Read the model definition and answer for the solid it produces. Units are mm, in the model's axes. Face numbers are marked on the shaded views. A direction names the side the tool comes from. Round coordinates to 2 decimals unless told otherwise and drop trailing zeros. Write each loop counter-clockwise with the first axis right and the second up, starting at its lowest first coordinate (ties: lowest second). Pieces come first, ordered by that corner, then holes.
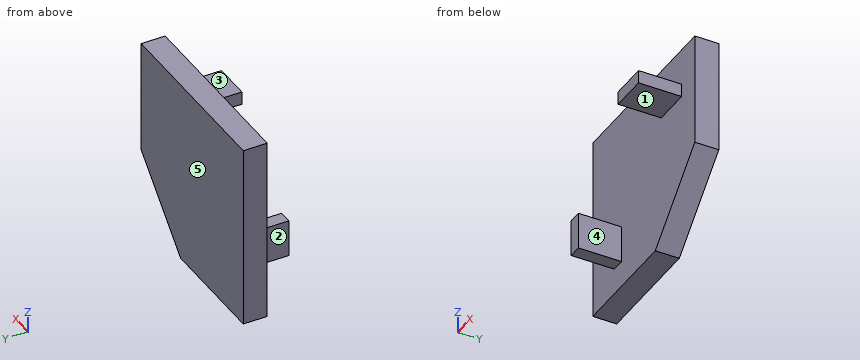
from build123d import *

# Parameters (mm, degrees)
SKETCH1_W           = 19.685
SKETCH1_H           = 19.685
BOSS_EXTRUDE1_DEPTH = 2.54
SKETCH3_W           = 1.397
SKETCH3_H           = 3.937
SKETCH3_W_2         = 3.937
SKETCH3_H_2         = 1.397
BOSS_EXTRUDE2_DEPTH = 4.572
CHAMFER1_SIZE       = 7.62


with BuildPart() as part:
    # Sketch1 → Boss-Extrude1 (new body)
    with BuildSketch(Plane(origin=(0, 0, 0), x_dir=(1, 0, 0), z_dir=(0, 1, 0))):
        Rectangle(SKETCH1_W, SKETCH1_H)
    extrude(amount=BOSS_EXTRUDE1_DEPTH)

    # Sketch3 → Boss-Extrude2 (add)
    with BuildSketch(Plane.XZ):
        with Locations((-4.98475, -5.08)):
            Rectangle(SKETCH3_W, SKETCH3_H)
        with Locations((5.334, 5.23748)):
            Rectangle(SKETCH3_W_2, SKETCH3_H_2)
    extrude(amount=BOSS_EXTRUDE2_DEPTH)

    # Chamfer1
    chamfer1_edges = [part.edges().sort_by_distance(p)[0] for p in [
        (9.8425, 1.27, -9.8425),
    ]]
    chamfer(chamfer1_edges, length=CHAMFER1_SIZE)


solid = part.part
Q1. Straight lines are drawn through the part: probe 1 along Y at (x, z) = (2, -9); probe 2 along X at (y, z) = (-2.75, -4.75); probe 3 along Z at (x, y) = (7, -3). For each, find the intervals that lie inside material, in ascending order.
Verdict:
probe 1: y = 0 to 2.54
probe 2: x = -5.68 to -4.29
probe 3: z = 4.54 to 5.94
Q2. Flat-ended cylindrical pins translate along their axes: pin 1 Ø3 at (y, z) = (-3, -5.5) entering from +X; pin 2 Ø1.1 at (y, z) = (-2, 5) entering from +X; pin 3 Ø6 at (x, z) = (-3, 4) entering from -Y. Find the tip coordinate at first contact, or state that the pin passes through.
Verdict:
pin 1: stops at x = -4.29
pin 2: stops at x = 7.3
pin 3: stops at y = 0
Q3. Section B-B (x = -5) is taken. Determine the outline of the cut face in (y, z).
Verdict:
outline: (-4.57, -7.05) - (0, -7.05) - (0, -9.84) - (2.54, -9.84) - (2.54, 9.84) - (0, 9.84) - (0, -3.11) - (-4.57, -3.11) - close
Q4. Section A-A (y = -0.25) is taken. Determine the outline of the cut face in (x, z).
Verdict:
outline: (-5.68, -7.05) - (-4.29, -7.05) - (-4.29, -3.11) - (-5.68, -3.11) - close; (3.37, 4.54) - (7.3, 4.54) - (7.3, 5.94) - (3.37, 5.94) - close
Q5. Section D-D (y = 1.25) is taken. Determine the outline of the cut face in (x, z).
Verdict:
outline: (-9.84, -9.84) - (2.22, -9.84) - (9.84, -2.22) - (9.84, 9.84) - (-9.84, 9.84) - close
Q6. Which of the six approach directions +Z, -Z, +X, -X, +Y, -Y give full straight-line access (tool end or side, diameter ignored) to the marked faces 1, 2, 3, 4 and 5?
Verdict:
face 1: -Z, +X, -X, -Y
face 2: +Z, -Z, -X, -Y
face 3: +Z, +X, -X, -Y
face 4: +Z, -Z, +X, -Y
face 5: +Z, -Z, +X, -X, +Y
Q7. Section C-C (z = -3.5) is taken. Determine the outline of the cut face in (x, y) (1 decimal), then the cut area to 3 significant figures.
Verdict:
outline: (-9.8, 0) - (-5.7, 0) - (-5.7, -4.6) - (-4.3, -4.6) - (-4.3, 0) - (8.6, 0) - (8.6, 2.5) - (-9.8, 2.5) - close
area: 53.1 mm2
